Could you check a few things on this model? Use its own coordinates, in mm. A direction names the side the tool comes from. Coordinates: 2 decimals unless noted, no trailing zeros. Write each loop counter-clockwise with the first axis right and the second up, starting at its lowest first coordinate (ties: lowest second). Pieces come first, ordered by that corner, then holes.
```python
from build123d import *

# Parameters (mm, degrees)
F0_W     = 39.9
F0_H     = 20.9
F1_DEPTH = 0.8
F3_DEPTH = 2.4
F4_SIZE  = 1.5


with BuildPart() as f1:
    # F0 (on Top) → F1 (new body)
    with BuildSketch(Plane.XY):
        Rectangle(F0_W, F0_H)
    extrude(amount=F1_DEPTH)

    # F2 (on face) → F3 (join)
    with BuildSketch(Plane.XY.offset(0.8)):
        Polygon((-12, -10), (-11.2, -10), (-11.2, -3.8), (1, -3.8), (1, -10), (1.8, -10), (1.8, -3.8), (19.5, -3.8), (19.5, -3), (1.8, -3), (1.8, 10), (1, 10), (1, -3), (-11.2, -3), (-11.2, 10), (-12, 10), align=None)
    extrude(amount=F3_DEPTH)

    # F4
    f4_edges = [f1.edges().sort_by_distance(p)[0] for p in [
        (-11.6, -10, 3.2),
        (1.4, -10, 3.2),
        (-11.6, 10, 3.2),
        (1.4, 10, 3.2),
        (19.5, -3.4, 3.2),
    ]]
    chamfer(f4_edges, length=F4_SIZE)


solid = f1.part
```
1. On a 3-axis mill with a long thin cutter (end or side, diameter ignored), from which of +Z, -Z, +X, -X, +Y, -Y can I reach the whole of each face in a straight line? I mean faces 4 (the face through (-12, 0, 2)), 5 (the face through (11, -3.8, 2)), 6 (the face through (1.8, 3, 2)), 7 (the face through (-5, -3, 2)). Say none if no direction works.
Verdict:
face 4: +Z, -X, +Y, -Y
face 5: +Z, +X, -Y
face 6: +Z, +X, +Y
face 7: +Z, +Y
2. If we mould it in two halves opening along X, with no side actions, what happens to faces 1 (the face through (-11.6, -9.2, 2.5)), 2 (the face through (1, -7, 2)), 3 (the face through (1.8, -7, 2))? For each: pulls with the +X half, pulls with the -X half, needs draft (parallel to the pull), parting line crosses it, or undercut.
Verdict:
face 1: needs draft
face 2: undercut
face 3: pulls with the +X half
3. I want a section at C-C on y = 5.5. Please give me the cut outline in (x, z), plus the area to 3 significant figures.
Verdict:
outline: (-19.95, 0) - (19.95, 0) - (19.95, 0.8) - (1.8, 0.8) - (1.8, 3.2) - (1, 3.2) - (1, 0.8) - (-11.2, 0.8) - (-11.2, 3.2) - (-12, 3.2) - (-12, 0.8) - (-19.95, 0.8) - close
area: 35.8 mm2
4. Please list where these lines run through material, in increasing order: line 1 along X through (y, z) = (-5, 2.3); line 2 along Z through (x, y) = (-17, 1.75); line 3 along Y through (x, z) = (-0.5, 2.2).
Verdict:
line 1: x = -12 to -11.2, 1 to 1.8
line 2: z = 0 to 0.8
line 3: y = -3.8 to -3
5. I want a section at B-B on x = 9. Please give me the cut outline in (y, z), plus the area to 3 significant figures.
Verdict:
outline: (-10.45, 0) - (10.45, 0) - (10.45, 0.8) - (-3, 0.8) - (-3, 3.2) - (-3.8, 3.2) - (-3.8, 0.8) - (-10.45, 0.8) - close
area: 18.6 mm2
6. I want a section at A-A on z = 1.2. Please give me the cut outline in (x, y).
Verdict:
outline: (-12, -10) - (-11.2, -10) - (-11.2, -3.8) - (1, -3.8) - (1, -10) - (1.8, -10) - (1.8, -3.8) - (19.5, -3.8) - (19.5, -3) - (1.8, -3) - (1.8, 10) - (1, 10) - (1, -3) - (-11.2, -3) - (-11.2, 10) - (-12, 10) - close
7. For pin 1 (1.9 mm diameter, centred on y = -7.5, z = 2.5, fed in from +X); pin 2 (1.9 mm diameter, centred on y = 6, z = 2, fed in from -X); pin 3 (0.6 mm diameter, centred on x = -11.5, z = 1.5, fed in from -Y), each with a flat end and sliding along its axis, tell me the tip position at first contact or that it passes through.
Verdict:
pin 1: stops at x = 1.8
pin 2: stops at x = -12
pin 3: stops at y = -10
8. I want a section at D-D on x = -16.5. Please give me the cut outline in (y, z).
Verdict:
outline: (-10.45, 0) - (10.45, 0) - (10.45, 0.8) - (-10.45, 0.8) - close
